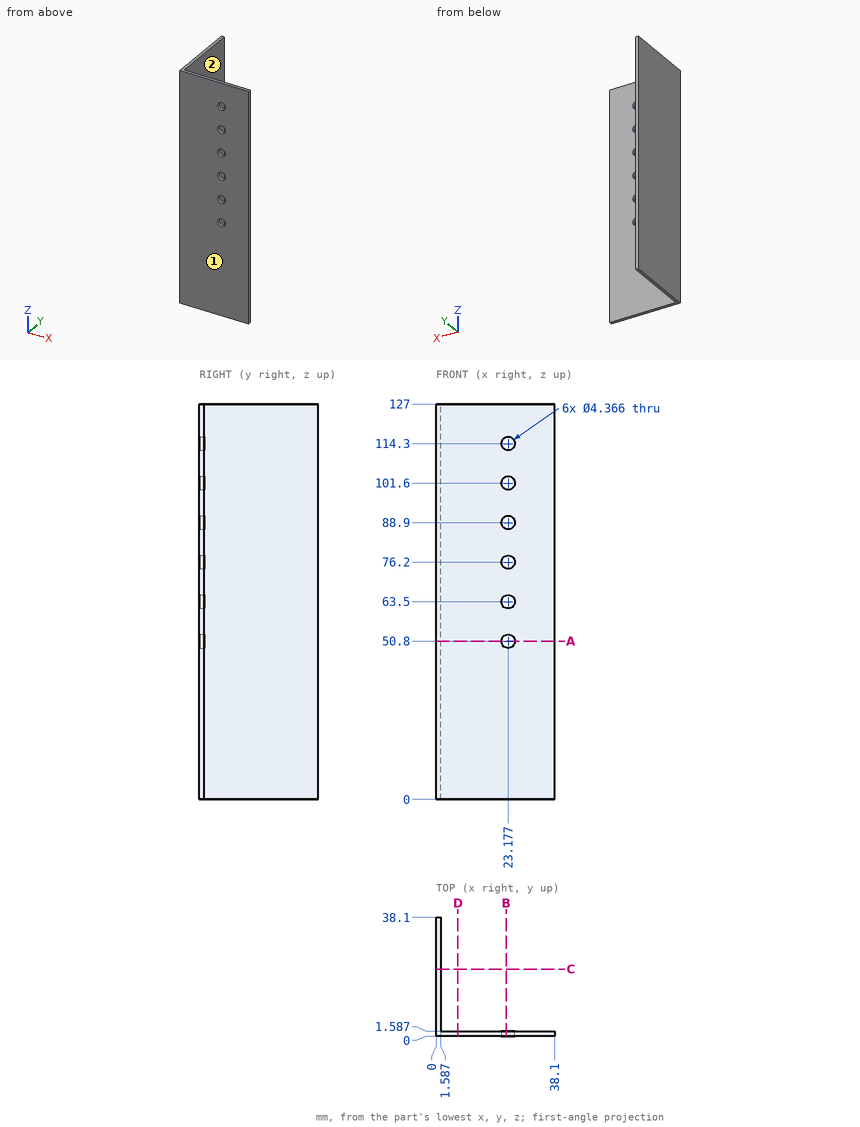
Geometry: see drawing. Coordinates: mm, zero at the bounding-box minimum. A direction names the side the tool comes from. Coordinates: 2 decimals unless noted, no trailing zeros. Loops run counter-clockwise (first coordinate to the right, second up) from the corner with the lowest first, then second, coordinate; pieces in that order, holes last. Notation, with made-up numbers: M 68,-6 L 122,-6 A21 cw 122,25 Z; hole C 72.5,87 d5. An arc over 180 degrees is marked long. Answer in a Markdown table with one row per item.
1. Section B-B, the plane x = 22.5. Output: boundary loops of the cut face in (y, z) (1 decimal).
Response:
| item | result |
|---|---|
| outline | M 0,0 L 1.6,0 L 1.6,48.7 L 0,48.7 Z; M 0,52.9 L 1.6,52.9 L 1.6,61.4 L 0,61.4 Z; M 0,65.6 L 1.6,65.6 L 1.6,74.1 L 0,74.1 Z; M 0,78.3 L 1.6,78.3 L 1.6,86.8 L 0,86.8 Z; M 0,91 L 1.6,91 L 1.6,99.5 L 0,99.5 Z; M 0,103.7 L 1.6,103.7 L 1.6,112.2 L 0,112.2 Z; M 0,116.4 L 1.6,116.4 L 1.6,127 L 0,127 Z |
2. Section A-A, the plane z = 50.8. Output: boundary loops of the cut face in (x, y) (1 decimal).
Response:
| item | result |
|---|---|
| outline | M 0,0 L 21,0 L 21,1.6 L 1.6,1.6 L 1.6,38.1 L 0,38.1 Z; M 25.4,0 L 38.1,0 L 38.1,1.6 L 25.4,1.6 Z |
3. Section C-C, the plane y = 21.5. Output: boundary loops of the cut face in (x, z).
Response:
| item | result |
|---|---|
| outline | M 0,0 L 1.59,0 L 1.59,127 L 0,127 Z |
4. Reachability of the marked faces 1 and 2 from +Z, -Z, +X, -X, +Y, -Y: full face, straight path, thin tool, end or side. Return the list, or none.
Response:
| item | result |
|---|---|
| face 1 | +Z, -Z, +X, -X, -Y |
| face 2 | +Z, -Z, +X, +Y |
5. First-contact query: pin 1 (18.5 mm diameter, centred on x = 13, z = 36.5, fed in from +Y); pin 2 (5.5 mm diameter, centred on x = 23.18, z = 76.2, fed in from -Y); pin 3 (4 mm diameter, centred on x = 23.18, z = 101.6, fed in from +Y); pin 4 (4 mm diameter, centred on y = 10.5, z = 31.5, fed in from +X). Flat tips, straight axial feed; report the tip coordinate or a pass-through.
Response:
| item | result |
|---|---|
| pin 1 | stops at y = 1.59 |
| pin 2 | stops at y = 0 |
| pin 3 | passes through |
| pin 4 | stops at x = 1.59 |
6. Material intervals for line 1 (X direction, y = 18, z = 110), sorted ascending.
Response:
| item | result |
|---|---|
| line 1 | x = 0 to 1.59 |
